Can you work these out from the model? Positions are in its coordinate system, mm. Face numbers are marked on the shaded views. A direction names the side the tool comes from. Give positions to 0.01 mm unless a question says otherwise; leave off trailing zeros. Write each loop counter-clockwise with the first axis right and the second up, starting at its lowest first coordinate (ties: lowest second). Pieces come first, ordered by that corner, then holes.
1. Suppose I cut it at B-B (y = 19). Please give me the cut outline in (x, z).
2. Suppose I cut it at C-C (z = 0). Please give me the cut outline in (x, y).
3. If I drill on probe 1 along Y at (x, z) = (-27.85, 0); probe 2 along X at (y, z) = (21.5, -3.5); probe 3 along Z at (x, y) = (0, -0.7), over which ranges is the centre line in solid material (lowest first)?
4. Suppose I cut it at A-A (x = 0). Please give me the cut outline in (y, z).
5. On a 3-axis mill with a long thin cutter (end or side, diameter ignored), from which of +Z, -Z, +X, -X, +Y, -Y can I reach the whole of each face in a straight line? I mean the marked faces 1 and 2. Say none if no direction works.
6. I'm going to push flat-ended pins straight in: pin 1 (3 mm diameter, centred on x = 0, z = 12.5, fed in from +Y); pin 2 (17 mm diameter, centred on x = -7.5, z = -3.5, fed in from +Y); pin 3 (1.7 mm diameter, centred on y = 4, z = 0, fed in from -X). Where does each tip first touch, or does it pass through?
7. Suppose I cut it at D-D (z = 7.5). Please give me the cut outline in (x, y).
```python
from build123d import *

# Parameters (mm, degrees)
BOSS_EXTRUDE1_DEPTH = 10
FILLET1_R           = 7
SKETCH2_R           = 1.45
SKETCH2_R_2         = 3.75
CUT_EXTRUDE1_DEPTH  = 15
BOSS_EXTRUDE2_DEPTH = 2
FILLET3_R           = 3
SKETCH4_R           = 1.75
CUT_EXTRUDE2_DEPTH  = 3


with BuildPart() as part:
    # Sketch1 → Boss-Extrude1 (new body, symmetric)
    with BuildSketch(Plane.XY):
        Polygon((-27.5, 25), (-27.5, 0), (27.5, 0), (27.5, 25), (29.5, 25), (29.5, -2), (-29.5, -2), (-29.5, 25), align=None)
    extrude(amount=BOSS_EXTRUDE1_DEPTH, both=True)

    # Fillet1
    fillet1_edges = [part.edges().sort_by_distance(p)[0] for p in [
        (-28.5, 25, -10),
        (28.5, 25, 10),
        (-28.5, 25, 10),
        (28.5, 25, -10),
    ]]
    fillet(fillet1_edges, radius=FILLET1_R)

    # Sketch2 → Cut-Extrude1 (cut, symmetric)
    with BuildSketch(Plane(origin=(-27.5, 0, 0), x_dir=(0, 0, -1), z_dir=(1, 0, 0))):
        with Locations((0, 19)):
            Circle(SKETCH2_R)
        with Locations((7.5, 11.5)):
            Circle(SKETCH2_R)
        with Locations((0, 4)):
            Circle(SKETCH2_R)
        with Locations((-7.5, 11.5)):
            Circle(SKETCH2_R)
        with Locations((0, 11.5)):
            Circle(SKETCH2_R_2)
    extrude(amount=CUT_EXTRUDE1_DEPTH, both=True, mode=Mode.SUBTRACT)

    # Sketch3 → Boss-Extrude2 (add)
    with BuildSketch(Plane(origin=(0, 0, 0), x_dir=(1, 0, 0), z_dir=(0, 1, 0))):
        Polygon((-8.5, 10), (0, 18), (8.5, 10), align=None)
        Polygon((8.5, -10), (-8.5, -10), (0, -18), align=None)
    extrude(amount=-BOSS_EXTRUDE2_DEPTH)

    # Fillet3
    fillet3_edges = [part.edges().sort_by_distance(p)[0] for p in [
        (8.5, -1, -10),
        (-8.5, -1, -10),
        (0, -1, -18),
        (8.5, -1, 10),
        (0, -1, 18),
        (-8.5, -1, 10),
    ]]
    fillet(fillet3_edges, radius=FILLET3_R)

    # Sketch4 → Cut-Extrude2 (cut, through all)
    with BuildSketch(Plane(origin=(0, 0, 0), x_dir=(1, 0, 0), z_dir=(0, 1, 0))):
        with Locations((0, 12.5)):
            Circle(SKETCH4_R)
        with Locations((0, -12.5)):
            Circle(SKETCH4_R)
    extrude(amount=-CUT_EXTRUDE2_DEPTH, mode=Mode.SUBTRACT)


solid = part.part
```
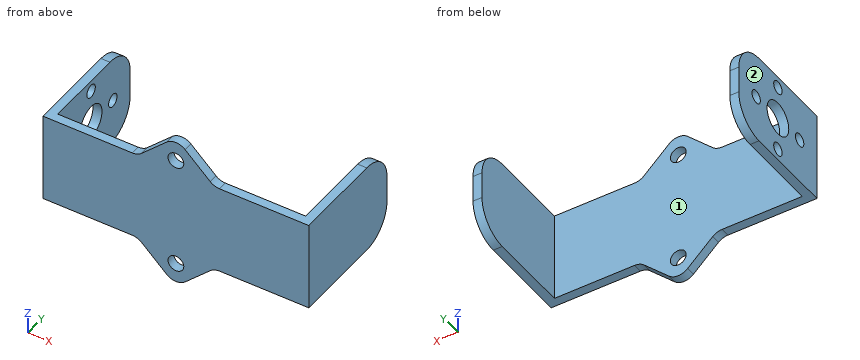
Checks:
1. outline: (-29.5, -9.93) - (-27.5, -9.93) - (-27.5, -1.45) - (-29.5, -1.45) - close; (-29.5, 1.45) - (-27.5, 1.45) - (-27.5, 9.93) - (-29.5, 9.93) - close; (27.5, -9.93) - (29.5, -9.93) - (29.5, 9.93) - (27.5, 9.93) - close
2. outline: (-29.5, -2) - (29.5, -2) - (29.5, 25) - (27.5, 25) - (27.5, 0) - (-27.5, 0) - (-27.5, 2.55) - (-29.5, 2.55) - close; (-29.5, 5.45) - (-27.5, 5.45) - (-27.5, 7.75) - (-29.5, 7.75) - close; (-29.5, 15.25) - (-27.5, 15.25) - (-27.5, 17.55) - (-29.5, 17.55) - close; (-29.5, 20.45) - (-27.5, 20.45) - (-27.5, 25) - (-29.5, 25) - close
3. probe 1: y = -2 to 2.55, 5.45 to 7.75, 15.25 to 17.55, 20.45 to 25
3. probe 2: x = -29.5 to -27.5, 27.5 to 29.5
3. probe 3: z = -16.88 to -14.25, -10.75 to 10.75, 14.25 to 16.88
4. outline: (-2, -16.88) - (0, -16.88) - (0, -14.25) - (-2, -14.25) - close; (-2, -10.75) - (0, -10.75) - (0, 10.75) - (-2, 10.75) - close; (-2, 14.25) - (0, 14.25) - (0, 16.88) - (-2, 16.88) - close
5. face 1: +Z, -Z, +Y
5. face 2: +Z, -Z, -X, +Y, -Y
6. pin 1: passes through
6. pin 2: stops at y = 0
6. pin 3: stops at x = 27.5
7. outline: (-29.5, -2) - (29.5, -2) - (29.5, 23.36) - (27.5, 23.36) - (27.5, 0) - (-27.5, 0) - (-27.5, 10.05) - (-29.5, 10.05) - close; (-29.5, 12.95) - (-27.5, 12.95) - (-27.5, 23.36) - (-29.5, 23.36) - close
